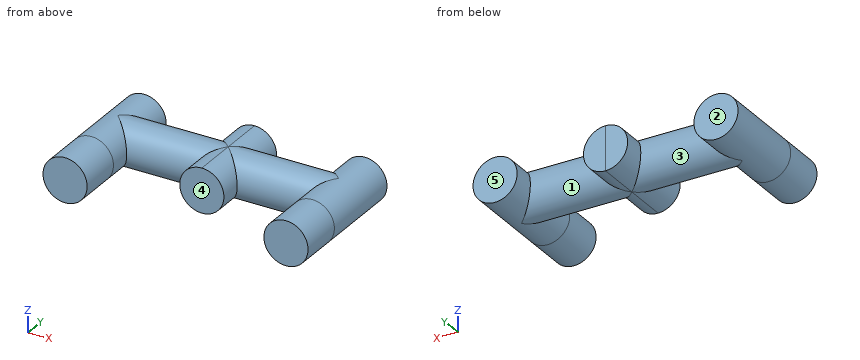
from build123d import *

# Parameters (mm, degrees)
SKETCH2_R           = 2.5
BOSS_EXTRUDE2_DEPTH = 10
SKETCH3_R           = 2.5
BOSS_EXTRUDE3_DEPTH = 12.5
BOSS_EXTRUDE4_DEPTH = 10
BOSS_EXTRUDE5_START = 5
SKETCH5_R           = 2.5
BOSS_EXTRUDE5_DEPTH = 5


with BuildPart() as part:
    # Sketch2 → Boss-Extrude2 (new body)
    with BuildSketch(Plane(origin=(0, 0, 0), x_dir=(1, 0, 0), z_dir=(0, 1, 0))):
        with Locations(Location((0, 0, 0), (0, 0, 270))):
            Circle(SKETCH2_R)
    boss_extrude2 = extrude(amount=BOSS_EXTRUDE2_DEPTH)

    # Sketch3 → Boss-Extrude3 (add)
    with BuildSketch(Plane(origin=(0, 0, 0), x_dir=(0, 0, -1), z_dir=(1, 0, 0))):
        with Locations((0, 5)):
            Circle(SKETCH3_R)
    boss_extrude3 = extrude(amount=BOSS_EXTRUDE3_DEPTH)

    # Sketch4 → Boss-Extrude4 (add)
    with BuildSketch(Plane(origin=(0, 0, 0), x_dir=(1, 0, 0), z_dir=(0, 1, 0))):
        with BuildLine():
            Line((12.5, 2.5), (12.5, -2.5))
            ThreePointArc((12.5, -2.5), (10, 0), (12.5, 2.5))
        make_face()
    boss_extrude4 = extrude(amount=BOSS_EXTRUDE4_DEPTH)

    # Mirror5: Boss-Extrude2, Boss-Extrude3, Boss-Extrude4 across plane
    add(boss_extrude2.mirror(Plane(origin=(12.5, 5, 0), x_dir=(0, 0, 1), z_dir=(1, 0, 0))))
    add(boss_extrude3.mirror(Plane(origin=(12.5, 5, 0), x_dir=(0, 0, 1), z_dir=(1, 0, 0))))
    add(boss_extrude4.mirror(Plane(origin=(12.5, 5, 0), x_dir=(0, 0, 1), z_dir=(1, 0, 0))))

    # Sketch5 → Boss-Extrude5 (add)
    with BuildSketch(Plane.XZ.offset(BOSS_EXTRUDE5_START)):
        with Locations(Location((0, 0, 0), (0, 0, 270))):
            Circle(SKETCH5_R)
        with Locations(Location((25, 0, 0), (0, 0, 270))):
            Circle(SKETCH5_R)
    extrude(amount=-BOSS_EXTRUDE5_DEPTH)


solid = part.part
For this review, take the finished solid that the model builds, in its own axes (mm). Face numbers are marked on the shaded views. A direction names the side the tool comes from. Round coordinates to 2 decimals unless told otherwise and drop trailing zeros. Loops run counter-clockwise (first coordinate to the right, second up) from the corner with the lowest first, then second, coordinate; pieces in that order, holes last. Notation, with made-up numbers: (40, 55.5) - (62, 55.5) arc R10 cw to (62, 67.5) - close; hole circle Ø9 at (58.5, -34). An arc over 180 degrees is marked (long way). Answer as CSV lines item,"result".
(1) Consider section D-D on y = 4. Give the boundary of the cut face in (x, z).
Checked values:
outline,"(1, -2.29) - (11.5, -2.29) arc R2.5 ccw to (13.5, -2.29) - (24, -2.29) arc R2.5 ccw (long way) to (24, 2.29) - (13.5, 2.29) arc R2.5 ccw to (11.5, 2.29) - (1, 2.29) arc R2.5 ccw (long way) to start"
(2) Insertion check: P1, Ø1, axis at x = 8, z = 0, coming from the -Y side; P2, Ø1, axis at x = 12.5, z = -0.5, coming from the -Y side; P3, Ø3, axis at x = 10.5, y = 3, coming from the +Z side. Each pin has a flat end and moves straight along its axis. Give the tip position at first contact, or say it passes through.
Checked values:
P1,"stops at y = 2.5"
P2,"stops at y = 0"
P3,"stops at z = 2.45"
(3) Tool access review of the marked faces 3, 4 and 5: name each direction out of +Z, -Z, +X, -X, +Y, -Y from which nothing blocks a thin tool from reaching the whole face with its end or side.
Checked values:
face 3,"none"
face 4,"+Z, -Z, -Y"
face 5,"+Z, -Z, +X, -X, +Y"
(4) Wall thickness on line 1 (X direction, y = 0.5, z = -0.05); line 2 (X direction, y = 3, z = -1.6); line 3 (X direction, y = -2.25, z = 0.1): over which ranges is each line inside the solid? List them lowest first.
Checked values:
line 1,"x = -2.5 to 2.5, 10 to 15, 22.5 to 27.5"
line 2,"x = -1.92 to 1.92, 10.58 to 14.42, 23.08 to 26.92"
line 3,"x = -2.5 to 2.5, 22.5 to 27.5"
(5) Mouldability with a two-part tool opening along X and no side actions: class the marked faces 1 and 2 as +X half, -X half, draft (parallel to the pull), parting line (faces both ways), or undercut.
Checked values:
face 1,"undercut"
face 2,"draft"
(6) Consider section A-A on z = 0. Give the boundary of the cut face in (x, y), then the cut area to 3 significant figures.
Checked values:
outline,"(-2.5, -5) - (2.5, -5) - (2.5, 2.5) - (10, 2.5) - (10, 0) - (15, 0) - (15, 2.5) - (22.5, 2.5) - (22.5, -5) - (27.5, -5) - (27.5, 10) - (22.5, 10) - (22.5, 7.5) - (15, 7.5) - (15, 10) - (10, 10) - (10, 7.5) - (2.5, 7.5) - (2.5, 10) - (-2.5, 10) - close"
area,"275 mm2"
(7) Consider section B-B on x = 1.5. Give the boundary of the cut face in (y, z).
Checked values:
outline,"(-5, -2) - (3.5, -2) arc R2.5 ccw to (6.5, -2) - (10, -2) - (10, 2) - (6.5, 2) arc R2.5 ccw to (3.5, 2) - (-5, 2) - close"
(8) Consider section C-C on y = 1.75. Give the boundary of the cut face in (x, z), then the cut area to 3 significant figures.
Checked values:
outline,"circle Ø5 at (0, 0); circle Ø5 at (12.5, 0); circle Ø5 at (25, 0)"
area,"58.9 mm2"
